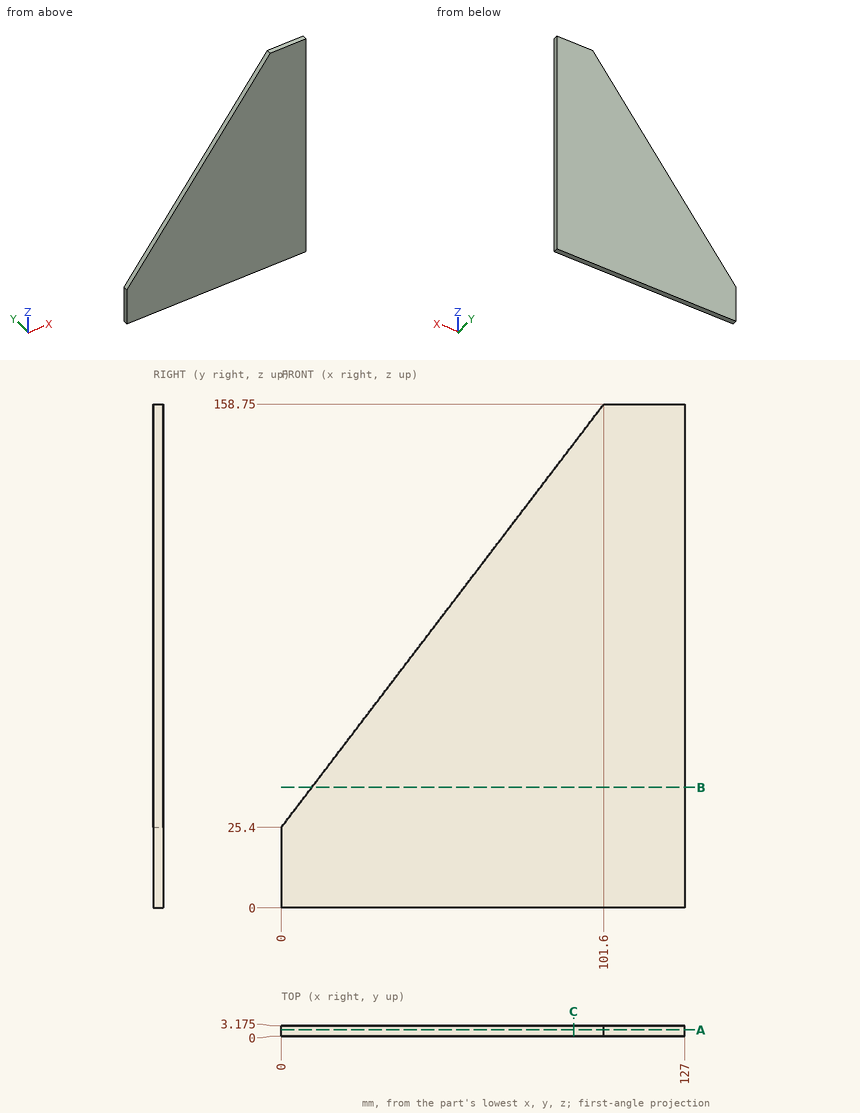
Job drawing, mm, ordinate dimensions from the low corner. One solid piece. Coordinates: 2 decimals unless noted, no trailing zeros. Loops run counter-clockwise (first coordinate to the right, second up) from the corner with the lowest first, then second, coordinate; pieces in that order, holes last. Notation, with made-up numbers: (-32.5, -34.75) - (20.5, -34.75) arc R21 ccw to (20.5, 1.25) - close; hole circle Ø9 at (28.5, 26). An arc over 180 degrees is marked (long way). Answer as a JSON object with one key per item and string values. Group by question number.
(1) Cut at B-B (z = 38). Give the cut face in (x, y) (3 decimals), then the cut area to 3 significant figures.
(2) Probe line 1 along X through (y, z) = (2.6, 142); line 2 along Z through (x, y) = (89.5, 1.05); line 3 along X through (y, z) = (2.65, 91). List the from-to ranges inside material, lowest first.
(3) Cut at A-A (y = 1.95). Give the cut face in (x, z), then the cut area to 3 significant figures.
(4) Cut at C-C (x = 92). Give the cut face in (y, z) (3 decimals), then the cut area to 3 significant figures.
Geometry says:
{
 "1": {"outline": "(9.6, 0) - (127, 0) - (127, 3.175) - (9.6, 3.175) - close", "area": "373 mm^2"},
 "2": {"line 1": "x = 88.84 to 127", "line 2": "z = 0 to 142.87", "line 3": "x = 49.98 to 127"},
 "3": {"outline": "(0, 0) - (127, 0) - (127, 158.75) - (101.6, 158.75) - (0, 25.4) - close", "area": "13,400 mm^2"},
 "4": {"outline": "(0, 0) - (3.175, 0) - (3.175, 146.15) - (0, 146.15) - close", "area": "464 mm^2"}
}
